from build123d import *

# Parameters (mm, degrees)
SKETCH_W        = 43
SKETCH_H        = 43
PAD_DEPTH       = 29
SKETCH001_W     = 41
SKETCH001_H     = 41
POCKET_DEPTH    = 28
SKETCH002_W     = 5
SKETCH002_H     = 5
PAD001_DEPTH    = 12
SKETCH003_R     = 0.625
POCKET001_DEPTH = 10
SKETCH004_W     = 26.5
SKETCH004_H     = 16
POCKET002_DEPTH = 1
SKETCH005_W     = 10
SKETCH005_H     = 5
SKETCH005_W_2   = 17
SKETCH005_H_2   = 4.5
POCKET003_DEPTH = 1
SKETCH006_W     = 2
SKETCH006_H     = 7
POCKET004_DEPTH = 1
FILLET_R        = 1
FILLET001_R     = 1
SKETCH007_W     = 7
SKETCH007_H     = 2
POCKET005_DEPTH = 1


with BuildPart() as part:
    # Sketch → Pad (new body)
    with BuildSketch(Plane.XY):
        Rectangle(SKETCH_W, SKETCH_H)
    extrude(amount=PAD_DEPTH)

    # Sketch001 (on Face6 of Pad) → Pocket (cut)
    with BuildSketch(Plane.XY.offset(29)):
        Rectangle(SKETCH001_W, SKETCH001_H)
    extrude(amount=-POCKET_DEPTH, mode=Mode.SUBTRACT)

    # Sketch002 (on Face11 of Pocket) → Pad001 (join)
    with BuildSketch(Plane.XY.offset(1)):
        with Locations((-18, 18)):
            Rectangle(SKETCH002_W, SKETCH002_H)
        with Locations((18, 18)):
            Rectangle(SKETCH002_W, SKETCH002_H)
        with Locations((-18, -18)):
            Rectangle(SKETCH002_W, SKETCH002_H)
        with Locations((18, -18)):
            Rectangle(SKETCH002_W, SKETCH002_H)
    extrude(amount=PAD001_DEPTH)

    # Sketch003 (on DatumPlane) → Pocket001 (cut)
    with BuildSketch(Plane.XY.offset(13)):
        with Locations((-17.7, 17.7)):
            Circle(SKETCH003_R)
        with Locations((17.7, 17.7)):
            Circle(SKETCH003_R)
        with Locations((-17.7, -17.7)):
            Circle(SKETCH003_R)
        with Locations((17.7, -17.7)):
            Circle(SKETCH003_R)
    extrude(amount=-POCKET001_DEPTH, mode=Mode.SUBTRACT)

    # Sketch004 (on Face6 of Pocket001) → Pocket002 (cut)
    with BuildSketch(Plane.XZ.offset(21.5)):
        with Locations((1.75, 21.5)):
            Rectangle(SKETCH004_W, SKETCH004_H)
    extrude(amount=-POCKET002_DEPTH, mode=Mode.SUBTRACT)

    # Sketch005 (on Face1 of Pocket002) → Pocket003 (cut)
    with BuildSketch(Plane(origin=(0, 21.5, 0), x_dir=(-1, 0, 0), z_dir=(0, 1, 0))):
        with Locations((-10.3, 17)):
            Rectangle(SKETCH005_W, SKETCH005_H)
        with Locations((7.2, 16.75)):
            Rectangle(SKETCH005_W_2, SKETCH005_H_2)
    extrude(amount=-POCKET003_DEPTH, mode=Mode.SUBTRACT)

    # Sketch006 (on Face3 of Pocket003) → Pocket004 (cut)
    with BuildSketch(Plane(origin=(0, 0, 0), x_dir=(1, 0, 0), z_dir=(0, 0, -1))):
        with Locations((13.5, -11)):
            Rectangle(SKETCH006_W, SKETCH006_H)
        with Locations((13.5, -2)):
            Rectangle(SKETCH006_W, SKETCH006_H)
        with Locations((9.5, -11)):
            Rectangle(SKETCH006_W, SKETCH006_H)
        with Locations((9.5, -2)):
            Rectangle(SKETCH006_W, SKETCH006_H)
        with Locations((5.5, -2)):
            Rectangle(SKETCH006_W, SKETCH006_H)
        with Locations((5.5, -11)):
            Rectangle(SKETCH006_W, SKETCH006_H)
        with Locations((1.5, -2)):
            Rectangle(SKETCH006_W, SKETCH006_H)
        with Locations((1.5, -11)):
            Rectangle(SKETCH006_W, SKETCH006_H)
        with Locations((-2.5, -2)):
            Rectangle(SKETCH006_W, SKETCH006_H)
        with Locations((-2.5, -11)):
            Rectangle(SKETCH006_W, SKETCH006_H)
    extrude(amount=-POCKET004_DEPTH, mode=Mode.SUBTRACT)

    # Fillet
    fillet_edges = [part.edges().sort_by_distance(p)[0] for p in [
        (-21.5, -21.5, 14.5),
        (21.5, -21.5, 14.5),
        (21.5, 21.5, 14.5),
        (-21.5, 21.5, 14.5),
    ]]
    fillet(fillet_edges, radius=FILLET_R)

    # Fillet001
    fillet001_edges = [part.edges().sort_by_distance(p)[0] for p in [
        (21.5, 0, 0),
        (0, -21.5, 0),
        (0, 21.5, 0),
        (-21.5, 0, 0),
    ]]
    fillet(fillet001_edges, radius=FILLET001_R)

    # Sketch007 (on Face22 of Fillet001) → Pocket005 (cut)
    with BuildSketch(Plane.YZ.offset(21.5)):
        with Locations((2, 10)):
            Rectangle(SKETCH007_W, SKETCH007_H)
        with Locations((11, 10)):
            Rectangle(SKETCH007_W, SKETCH007_H)
        with Locations((2, 7)):
            Rectangle(SKETCH007_W, SKETCH007_H)
        with Locations((11, 7)):
            Rectangle(SKETCH007_W, SKETCH007_H)
        with Locations((2, 4)):
            Rectangle(SKETCH007_W, SKETCH007_H)
        with Locations((11, 4)):
            Rectangle(SKETCH007_W, SKETCH007_H)
    extrude(amount=-POCKET005_DEPTH, mode=Mode.SUBTRACT)


solid = part.part
Read the model definition and answer for the solid it produces. Units are mm, in the model's axes. A direction names the side the tool comes from. Coordinates: 2 decimals unless noted, no trailing zeros. Write each loop counter-clockwise with the first axis right and the second up, starting at its lowest first coordinate (ties: lowest second). Pieces come first, ordered by that corner, then holes. Notation, with made-up numbers: M 88.5,88.25 L 96.5,88.25 A34 cw 96.5,121.25 Z; hole C 7.5,18 d9. An arc over 180 degrees is marked long. Use a Markdown table: item, result.
Q1. Which of the six approach directions +Z, -Z, +X, -X, +Y, -Y give full straight-line access (tool end or side, diameter ignored) to faces 5 (the face through (-21.5, 0, 15)), 6 (the face through (-15.5, -18, 7))?
Answer block:
| item | result |
|---|---|
| face 5 | +Z, -Z, -X, +Y, -Y |
| face 6 | +Z |
Q2. The part is cut by section A-A, the plane z = 2.25. Write down the section's boundary in (x, y), then the cut area to 3 significant figures.
Answer block:
| item | result |
|---|---|
| outline | M -21.5,-20.5 A1 ccw -20.5,-21.5 L 20.5,-21.5 A1 ccw 21.5,-20.5 L 21.5,20.5 A1 ccw 20.5,21.5 L -20.5,21.5 A1 ccw -21.5,20.5 Z; hole M -20.5,-15.5 L -15.5,-15.5 L -15.5,-20.5 L 15.5,-20.5 L 15.5,-15.5 L 20.5,-15.5 L 20.5,15.5 L 15.5,15.5 L 15.5,20.5 L -15.5,20.5 L -15.5,15.5 L -20.5,15.5 Z |
| area | 267 mm2 |
Q3. Straight lines are drawn through the part: L1, parallel to Y at x = -17.7, z = 7 (3 decimals); L2, parallel to Y at x = 8.5, z = 2.5. For each, find the intervals that lie inside material, in ascending order. Write a range as [from, to].
Answer block:
| item | result |
|---|---|
| L1 | y = [-21.5, -18.325], [-17.075, -15.5], [15.5, 17.075], [18.325, 21.5] |
| L2 | y = [-21.5, -20.5], [20.5, 21.5] |
Q4. Each of these flat-tipped pins is pushed along its axis until it touches: pin 1 Ø0.5 at (x, z) = (21, 9.5) entering from -Y; pin 2 Ø0.5 at (x, y) = (21, 1.5) entering from -Z; pin 3 Ø3 at (x, z) = (-8.5, 19.5) entering from -Y. Where does it stop, or does it pass through?
Answer block:
| item | result |
|---|---|
| pin 1 | stops at y = -21.47 |
| pin 2 | stops at z = 0.03 |
| pin 3 | stops at y = 20.5 |
Q5. The part is cut by section B-B, the plane x = -17.7. Write down the section's boundary in (y, z) (3 decimals), then the cut area to 3 significant figures.
Answer block:
| item | result |
|---|---|
| outline | M -21.5,1 A1 ccw -20.5,0 L 20.5,0 A1 ccw 21.5,1 L 21.5,29 L 20.5,29 L 20.5,13 L 18.325,13 L 18.325,3 L 17.075,3 L 17.075,13 L 15.5,13 L 15.5,1 L -15.5,1 L -15.5,13 L -17.075,13 L -17.075,3 L -18.325,3 L -18.325,13 L -20.5,13 L -20.5,29 L -21.5,29 Z |
| area | 194 mm2 |
Q6. Determine the mould class of faces 1 (the face through (19, 18, 13)), 2 (the face through (0, 21.5, 12)), 3 (the face through (21.5, 0, 15)), 4 (the face through (19, -18, 13)) for opening direction Y: released by +Y, released by -Y, zero draft, split by the parting line, or undercut.
Answer block:
| item | result |
|---|---|
| face 1 | undercut |
| face 2 | released by +Y |
| face 3 | zero draft |
| face 4 | undercut |
Q7. The part is cut by section D-D, the plane z = 26.25. Write down the section's boundary in (x, y).
Answer block:
| item | result |
|---|---|
| outline | M -21.5,-20.5 A1 ccw -20.5,-21.5 L -11.5,-21.5 L -11.5,-20.5 L -20.5,-20.5 L -20.5,20.5 L 20.5,20.5 L 20.5,-20.5 L 15,-20.5 L 15,-21.5 L 20.5,-21.5 A1 ccw 21.5,-20.5 L 21.5,20.5 A1 ccw 20.5,21.5 L -20.5,21.5 A1 ccw -21.5,20.5 Z |
